Check sheet for the modelled part. Datum: model origin and axes. Units: mm. A direction names the side the tool comes from. Give positions to 0.01 mm unless a question says otherwise; leave off trailing zeros. Order: outer loops, then holes, each group sorted by start corner. A loop starts at its lowest first (then second) coordinate and runs counter-clockwise, first axis right, second up. Notation, with made-up numbers: (63, 67) - (71, 67) arc R19 ccw to (71, 77) - close; hole circle Ø11 at (67, 67). An arc over 180 degrees is marked (long way). Answer in a Markdown table with one row per item.
Autodesk Inventor part; units mm, degrees
ref_plane "YZ Plane" through (0, 0, 0) normal (1, 0, 0) x (0, 1, 0)
ref_plane "XZ Plane" through (0, 0, 0) normal (0, 1, 0) x (-1, 0, 0)
ref_plane "XY Plane" through (0, 0, 0) normal (0, 0, 1) x (1, 0, 0)
sketch "Boceto1" plane through (0, 0, 0) normal (0, 0, 1) x (1, 0, 0)
  line L0 (25, -3) -> (15, -3)
  line L1 (25, -3) -> (25, -6)
  line L2 (15, -6) -> (15, -3)
  line L3 (0, 0) -> (0, -3)
  line L4 (40, -6) -> (40, -3)
  line L5 (28.1623, -51) -> (8.1623, -51)
  line L6 (0, -6) -> (15, -6)
  line L7 (25, -6) -> (40, -6)
  line L8 (0, -6) -> (0, -51)
  line L9 (0, -51) -> (40, -51)
  line L10 (40, -51) -> (40, -6)
  line L11 (40, -6) -> (25, -6)
  line L12 (15, -6) -> (0, -6)
  point P0 (0, 0)
extrude "Extrusión1" add sketch "Boceto1" along normal blind 3
sketch "Boceto2" plane through (0, 0, 3) normal (0, 0, 1) x (1, 0, 0)
  line L0 (25, -6) -> (25, -3)
  line L1 (25, -3) -> (15, -3)
  line L2 (15, -3) -> (15, -6)
  line L3 (15, -6) -> (0, -6)
  line L4 (0, -6) -> (0, -51)
  line L5 (0, -51) -> (40, -51)
  line L6 (40, -51) -> (40, -6)
  line L7 (40, -6) -> (25, -6)
  line L8 (40, -51) -> (40, -6)
  line L9 (0, -51) -> (40, -51)
  line L10 (0, -6) -> (0, -51)
  line L11 (15, -6) -> (0, -6)
  line L12 (15, -3) -> (15, -6)
  line L13 (40, -6) -> (25, -6)
  line L14 (25, -6) -> (25, -3)
  line L15 (25, -3) -> (15, -3)
  line L16 (9.8382, -32) -> (1.6623, -32)
  line L17 (9.8382, -31) -> (1.6623, -31)
  line L18 (1.1623, 19) -> (1.1623, 20)
  line L19 (10.1623, -31) -> (10.1623, -32)
  line L20 (9.8382, -30) -> (1.6623, -30)
  line L21 (9.8382, -29) -> (1.6623, -29)
  line L22 (1.1623, 21) -> (1.1623, 22)
  line L23 (10.1623, -29) -> (10.1623, -30)
  line L24 (9.8382, -25) -> (1.6623, -25)
  line L25 (1.1623, 25) -> (1.1623, 26)
  line L26 (9.8382, -26) -> (9.8382, -25)
  line L27 (0, -34) -> (12.1623, -34)
  line L28 (12.1623, -34) -> (12.1623, -23)
  line L29 (12.1623, -23) -> (0, -23)
  line L30 (0, -23) -> (0, -34)
  point P0 (0, 0)
extrude "Extrusión2" cut sketch "Boceto2" against normal blind 3 contours L4 L29 L28 L27
sketch "Boceto3" plane through (0, 0, 3) normal (0, 0, 1) x (1, 0, 0)
  line L0 (12.1623, -34) -> (0, -34)
  line L1 (0, -34) -> (0, -51)
  line L2 (0, -51) -> (40, -51)
  line L3 (40, -51) -> (40, -6)
  line L4 (40, -6) -> (25, -6)
  line L5 (25, -6) -> (25, -3)
  line L6 (25, -3) -> (15, -3)
  line L7 (15, -3) -> (15, -6)
  line L8 (15, -6) -> (0, -6)
  line L9 (0, -6) -> (0, -23)
  line L10 (0, -23) -> (12.1623, -23)
  line L11 (12.1623, -23) -> (12.1623, -34)
  line L12 (12.1623, -34) -> (13.1623, -34)
  line L13 (13.1623, -34) -> (15.1623, -34)
  line L14 (15.1623, -34) -> (-10.6091, -34)
  line L15 (-10.6091, -34) -> (-10.6091, -23)
  line L16 (-10.6091, -23) -> (15.1623, -23)
  line L17 (15.1623, -23) -> (15.1623, -34)
  point P0 (0, 0)
  dimension "d4" = 1
  dimension "d5" = 2
extrude "Extrusión3" cut sketch "Boceto3" against normal blind 3 contours L0 L14 L15 L16 L10 L11 | L11 L16 L17 L13 L12
properties part number "acople 3" material "Madera (nogal)"
(1) Gauge pin test, flat ends, axial feed: P1, Ø1.5, axis at x = 11, z = 1.5, coming from the +Y side; P2, Ø1.5, axis at x = 5.5, y = -11.5, coming from the -Z side; P3, Ø0.9, axis at y = -4, z = 1.5, coming from the +X side. Record the tip position at first contact, or that the pin passes through.
Geometry says:
| item | result |
|---|---|
| P1 | y = -6 |
| P2 | z = 0 |
| P3 | x = 25 |
(2) Cross-section at B-B, the plane z = 2.4. Record the cut outline in (x, y).
Geometry says:
| item | result |
|---|---|
| outline | (0, -51) - (40, -51) - (40, -6) - (25, -6) - (25, -3) - (15, -3) - (15, -6) - (0, -6) - (0, -23) - (15.16, -23) - (15.16, -34) - (0, -34) - close |
(3) Cross-section at D-D, the plane y = -29.5. Record the cut outline in (x, z).
Geometry says:
| item | result |
|---|---|
| outline | (15.16, 0) - (40, 0) - (40, 3) - (15.16, 3) - close |
(4) Access from +Z, -Z, +X, -X, +Y, -Y to the whole of each face (thin tool, end or side, straight path). Record for faces 4 (the flat face through (25, -4, 1)), 5 (the flat face through (7, -34, 2)), 6 (the flat face through (7, -6, 1)).
Geometry says:
| item | result |
|---|---|
| face 4 | +Z, -Z, +X, +Y |
| face 5 | +Z, -Z, -X |
| face 6 | +Z, -Z, -X, +Y |
(5) Cross-section at C-C, the plane x = 27. Record the cut outline in (y, z), then the cut area to 3 significant figures.
Geometry says:
| item | result |
|---|---|
| outline | (-51, 0) - (-6, 0) - (-6, 3) - (-51, 3) - close |
| area | 135 mm² |
(6) Cross-section at A-A, the plane x = 14. Record the cut outline in (y, z), then the cut area to 3 significant figures.
Geometry says:
| item | result |
|---|---|
| outline | (-51, 0) - (-34, 0) - (-34, 3) - (-51, 3) - close; (-23, 0) - (-6, 0) - (-6, 3) - (-23, 3) - close |
| area | 102 mm² |
(7) Mould release check, pull along Y, two halves, no side actions. Record for faces 1 (the flat face through (15, -5, 1)), 2 (the flat face through (32, -6, 1)), 3 (the flat face through (7, -23, 2)): pulls with the +Y half, pulls with the -Y half, needs draft (parallel to the pull), parting line crosses it, or undercut.
Geometry says:
| item | result |
|---|---|
| face 1 | needs draft |
| face 2 | pulls with the +Y half |
| face 3 | undercut |
(8) Thickness scan on L1, parallel to Y at x = 13.5, z = 2.75; L2, parallel to Y at x = 25.5, z = 1.5. Record the ranges inside material, lowest first.
Geometry says:
| item | result |
|---|---|
| L1 | -51 to -34, -23 to -6 |
| L2 | -51 to -6 |
